Here's how the part is built. I have some questions about the finished solid (model axes, mm). A direction names the side the tool comes from. Coordinates: 2 decimals unless noted, no trailing zeros. Answer as CSV lines item,"result". Start each with the question number.
Q1. Suppose I cut it at A-A (z = 0.25). Count the separate pieces of the cut face and the enclosed holes in it, then the cut area to 3 significant figures.
Q2. For pin 1 Ø3.5 at (x, z) = (75, 1) entering from -Y; pin 2 Ø8 at (x, y) = (39, -26.5) entering from +Z; pin 3 Ø1.8 at (y, z) = (-27, 4) entering from +X; pin 4 Ø6 at (x, y) = (50.5, -38) entering from -Z, each with a flat end and sliding along its axis, tell me the tip position at first contact or that it passes through.
Q3. Thinking about a two-plate mould opening in Y: for faces 4 (the face through (48.665, -27.866, 5.967)), 5 (the face through (48, -27, 6.096)), 6 (the face through (23, 0, 0)), 7 (the face through (70.16, -21.91, 5.97)), which applies, released by +Y, released by -Y, zero draft, split by the parting line, or undercut?
Q4. For faces 1 (the face through (70.02, -9.88, 4.09)), 2 (the face through (2.54, -22, -4)), 3 (the face through (3.349, -3.525, -5.967)), which set-ups out of +Z, -Z, +X, -X, +Y, -Y let a thin tool reach every point of the face, with its end or its side?
Q5. I need wall thicknesses on line 1 (Y direction, x = 55, z = -3.25); line 2 (X direction, y = -31.5, z = 4.25); line 3 (Y direction, x = 32, z = -3). Which ranges of each line are inside material? Lowest first, please.
from build123d import *

# Parameters (mm, degrees)
SKETCH1_W           = 96.52
SKETCH1_H           = 44.45
BOSS_EXTRUDE1_DEPTH = 6.096
CUT_EXTRUDE1_REACH  = 108.961
SKETCH2_R           = 11.50874
CUT_EXTRUDE2_REACH  = 108.438
SKETCH3_R           = 3.3782
CUT_EXTRUDE3_REACH  = 108.961
SKETCH7_W           = 12.7635
SKETCH7_H           = 12.192
CUT_EXTRUDE5_DEPTH  = 104.946532487
FILLET1_R           = 11.43
SKETCH5_R           = 12.77874
CUT_EXTRUDE4_DEPTH  = 3.81
CHAMFER1_SIZE       = 0.254


with BuildPart() as part:
    # Sketch1 → Boss-Extrude1 (new, symmetric)
    with BuildSketch(Plane.XY):
        with Locations((48.26, -22.225)):
            Rectangle(SKETCH1_W, SKETCH1_H)
    extrude(amount=BOSS_EXTRUDE1_DEPTH, both=True)

    # Sketch2 → Cut-Extrude1 (cut, up to next)
    with BuildSketch(Plane.XY.offset(6.096), mode=Mode.PRIVATE) as cut_extrude1_sk1:
        with Locations((22.225, -22.225)):
            Circle(SKETCH2_R)
    cut_extrude1_tool1 = extrude(cut_extrude1_sk1.sketch, amount=-CUT_EXTRUDE1_REACH, mode=Mode.PRIVATE) & part.part
    add(cut_extrude1_tool1.solids().sort_by_distance((22.225, -22.225, 6.096))[0], mode=Mode.SUBTRACT)

    # Sketch3 → Cut-Extrude2 (cut, up to next)
    with BuildSketch(Plane(origin=(0, 0, 0), x_dir=(1, 0, 0), z_dir=(0, 1, 0)), mode=Mode.PRIVATE) as cut_extrude2_sk1:
        with Locations(Location((77.4065, -0.254, 0), (0, 0, 270))):
            Circle(SKETCH3_R)
    cut_extrude2_tool1 = extrude(cut_extrude2_sk1.sketch, amount=-CUT_EXTRUDE2_REACH, mode=Mode.PRIVATE) & part.part
    add(cut_extrude2_tool1.solids().sort_by_distance((77.4065, 0, 0.254))[0], mode=Mode.SUBTRACT)

    # Sketch4 → Cut-Extrude3 (cut, up to next)
    with BuildSketch(Plane.XY.offset(6.096), mode=Mode.PRIVATE) as cut_extrude3_sk1:
        with BuildLine():
            Line((48.895, 6.35), (96.52, 6.35))
            ThreePointArc((96.52, 6.35), (102.87, 0), (96.52, -6.35))
            Line((96.52, -6.35), (48.895, -6.35))
            ThreePointArc((48.895, -6.35), (42.545, 0), (48.895, 6.35))
        make_face()
    cut_extrude3_tool1 = extrude(cut_extrude3_sk1.sketch, amount=-CUT_EXTRUDE3_REACH, mode=Mode.PRIVATE) & part.part
    # Sketch4 → Cut-Extrude3 (cut, up to next)
    with BuildSketch(Plane.XY.offset(6.096), mode=Mode.PRIVATE) as cut_extrude3_sk2:
        with BuildLine():
            Line((45.72, -34.925), (45.72, -44.45))
            Line((45.72, -44.45), (55.245, -44.45))
            Line((55.245, -44.45), (96.52, -44.45))
            ThreePointArc((96.52, -44.45), (106.045, -34.925), (96.52, -25.4))
            Line((96.52, -25.4), (55.245, -25.4))
            ThreePointArc((55.245, -25.4), (48.509807909, -28.189807909), (45.72, -34.925))
        make_face()
    cut_extrude3_tool2 = extrude(cut_extrude3_sk2.sketch, amount=-CUT_EXTRUDE3_REACH, mode=Mode.PRIVATE) & part.part
    add(cut_extrude3_tool1.solids().sort_by_distance((72.7075, 0, 6.096))[0], mode=Mode.SUBTRACT)
    add(cut_extrude3_tool2.solids().sort_by_distance((75.382091, -35.05704, 6.096))[0], mode=Mode.SUBTRACT)

    # Sketch7 → Cut-Extrude5 (cut, through all)
    with BuildSketch(Plane(origin=(0, -6.35, 0), x_dir=(1, 0, 0), z_dir=(0, 1, 0))):
        with Locations((90.13825, 0)):
            Rectangle(SKETCH7_W, SKETCH7_H)
    extrude(amount=-CUT_EXTRUDE5_DEPTH, mode=Mode.SUBTRACT)

    # Fillet1
    fillet1_edges = [part.edges().sort_by_distance(p)[0] for p in [
        (42.545, 0, 0),
        (45.72, -44.45, 0),
        (0, -44.45, 0),
        (0, 0, 0),
    ]]
    fillet(fillet1_edges, radius=FILLET1_R)

    # Sketch5 → Cut-Extrude4 (cut)
    with BuildSketch(Plane.XY.offset(6.096)):
        with BuildLine():
            Line((71.0565, -12.3444), (71.0565, -19.4056))
            ThreePointArc((71.0565, -19.4056), (70.044729665, -21.848229665), (67.6021, -22.86))
            Line((67.6021, -22.86), (55.245, -22.86))
            ThreePointArc((55.245, -22.86), (47.110778659, -26.014406968), (43.229958807, -33.828181818))
            ThreePointArc((43.229958807, -33.828181818), (40.370407336, -39.585700129), (34.376770559, -41.91))
            Line((34.376770559, -41.91), (11.43, -41.91))
            ThreePointArc((11.43, -41.91), (5.143820715, -39.306179285), (2.54, -33.02))
            Line((2.54, -33.02), (2.54, -11.43))
            ThreePointArc((2.54, -11.43), (5.143820715, -5.143820715), (11.43, -2.54))
            Line((11.43, -2.54), (35.275767276, -2.54))
            ThreePointArc((35.275767276, -2.54), (39.032477938, -3.372753262), (42.085383638, -5.715))
            ThreePointArc((42.085383638, -5.715), (45.138289338, -8.057246738), (48.895, -8.89))
            Line((48.895, -8.89), (67.6021, -8.89))
            ThreePointArc((67.6021, -8.89), (70.044729665, -9.901770335), (71.0565, -12.3444))
        make_face()
        with Locations((22.225, -22.225)):
            Circle(SKETCH5_R, mode=Mode.SUBTRACT)
    cut_extrude4 = extrude(amount=-CUT_EXTRUDE4_DEPTH, mode=Mode.SUBTRACT)

    # Mirror3: Cut-Extrude4 across plane
    add(cut_extrude4.mirror(Plane.XY), mode=Mode.SUBTRACT)

    # Chamfer1
    chamfer1_edges = [part.edges().sort_by_distance(p)[0] for p in [
        (70.044729665, -21.848229665, 6.096),
        (71.0565, -15.875, 6.096),
        (70.044729665, -9.901770335, 6.096),
        (58.24855, -8.89, 6.096),
        (45.138289338, -8.057246738, 6.096),
        (39.032477938, -3.372753262, 6.096),
        (23.352883638, -2.54, 6.096),
        (5.143820715, -5.143820715, 6.096),
        (2.54, -22.225, 6.096),
        (5.143820715, -39.306179285, 6.096),
        (22.90338528, -41.91, 6.096),
        (40.370407336, -39.585700129, 6.096),
        (47.110778659, -26.014406968, 6.096),
        (61.42355, -22.86, 6.096),
        (10.71626, -22.225, 6.096),
        (70.044729665, -21.848229665, -6.096),
        (71.0565, -15.875, -6.096),
        (70.044729665, -9.901770335, -6.096),
        (58.24855, -8.89, -6.096),
        (45.138289338, -8.057246738, -6.096),
        (39.032477938, -3.372753262, -6.096),
        (23.352883638, -2.54, -6.096),
        (5.143820715, -5.143820715, -6.096),
        (2.54, -22.225, -6.096),
        (5.143820715, -39.306179285, -6.096),
        (22.90338528, -41.91, -6.096),
        (40.370407336, -39.585700129, -6.096),
        (47.110778659, -26.014406968, -6.096),
        (61.42355, -22.86, -6.096),
        (46.211635241, -5.755176242, -6.096),
        (66.32575, -6.35, 6.096),
        (69.50075, -25.4, -6.096),
        (48.82324631, -27.890321291, 6.096),
        (66.32575, -6.35, -6.096),
        (69.50075, -25.4, 6.096),
        (46.211635241, -5.755176242, 6.096),
        (23.352883638, 0, 6.096),
        (0, -22.225, 6.096),
        (22.90338528, -44.45, 6.096),
        (3.347769491, -3.347769491, 6.096),
        (3.347769491, -41.102230509, 6.096),
        (42.082874987, -41.461614451, 6.096),
        (40.105823841, -1.070682765, 6.096),
        (23.352883638, 0, -6.096),
        (48.82324631, -27.890321291, -6.096),
        (22.90338528, -44.45, -6.096),
        (0, -22.225, -6.096),
        (3.347769491, -3.347769491, -6.096),
        (3.347769491, -41.102230509, -6.096),
        (42.082874987, -41.461614451, -6.096),
        (40.105823841, -1.070682765, -6.096),
    ]]
    chamfer(chamfer1_edges, length=CHAMFER1_SIZE)


solid = part.part
Here are the results:
1,separate pieces,"2"
1,enclosed holes,"1"
1,area,"2,130 mm²"
2,pin 1,"stops at y = -25.4"
2,pin 2,"stops at z = 2.29"
2,pin 3,"stops at x = 51.66"
2,pin 4,"passes through"
3,face 4,"released by -Y"
3,face 5,"zero draft"
3,face 6,"released by +Y"
3,face 7,"undercut"
4,face 1,"+Z"
4,face 2,"-Z"
4,face 3,"-Z, -X, +Y"
5,line 1,"y = -25.4 to -22.86, -8.89 to -6.35"
5,line 2,"x = 0 to 2.54, 13.43 to 15.41, 29.04 to 31.02, 43.68 to 46.36"
5,line 3,"y = -44.45 to -41.91, -30.46 to -28.3, -16.15 to -13.99, -2.54 to 0"
